from build123d import *

# Parameters (mm, degrees)
F0_W     = 90
F0_H     = 60
F0_R     = 2.15
F1_DEPTH = 60
F2_R     = 1.5
F3_DEPTH = 60
F4_W     = 50
F4_H     = 50
F5_DEPTH = 90


with BuildPart() as f1:
    # F0 (on Top) → F1 (new body)
    with BuildSketch(Plane.XY):
        Rectangle(F0_W, F0_H)
        with Locations((-39.25, -13)):
            Circle(F0_R, mode=Mode.SUBTRACT)
        with Locations((-8.75, -13)):
            Circle(F0_R, mode=Mode.SUBTRACT)
        with Locations((8.75, -13)):
            Circle(F0_R, mode=Mode.SUBTRACT)
        with Locations((39.25, -13)):
            Circle(F0_R, mode=Mode.SUBTRACT)
        with Locations((-39.25, 13)):
            Circle(F0_R, mode=Mode.SUBTRACT)
        with Locations((-8.75, 13)):
            Circle(F0_R, mode=Mode.SUBTRACT)
        with Locations((8.75, 13)):
            Circle(F0_R, mode=Mode.SUBTRACT)
        with Locations((39.25, 13)):
            Circle(F0_R, mode=Mode.SUBTRACT)
    extrude(amount=-F1_DEPTH)

    # F2 (on face) → F3 (cut)
    with BuildSketch(Plane.XY):
        Circle(F2_R)
    extrude(amount=-F3_DEPTH, mode=Mode.SUBTRACT)

    # F4 (on face) → F5 (cut)
    with BuildSketch(Plane.YZ.offset(45)):
        with Locations((0, -30)):
            Rectangle(F4_W, F4_H)
    extrude(amount=-F5_DEPTH, mode=Mode.SUBTRACT)


solid = f1.part
Can you work these out from the model? Positions are in its coordinate system, mm. A direction names the side the tool comes from. Round coordinates to 2 decimals unless told otherwise and drop trailing zeros. Write each loop counter-clockwise with the first axis right and the second up, starting at its lowest first coordinate (ties: lowest second). Pieces come first, ordered by that corner, then holes. Notation, with made-up numbers: (35.5, -30.75) -> (93.5, -30.75) arc R12 ccw to (93.5, -26.75) -> close; hole circle Ø6 at (7, -34). An arc over 180 degrees is marked (long way). Use one line per item in the form item = value. Start each with the question number.
Q1. Imagine slicing it at D-D (y = 0). Please give me the cut outline in (x, z), then the cut area to 3 significant figures.
Q2. Imagine slicing it at B-B (x = 0). Please give me the cut outline in (y, z).
Q3. Which directions (+Z, -Z, +X, -X, +Y, -Y) give clear straight access to the entire face, cutting with the end or side of a thin tool? Please do faces 4 (the face through (1, 5, -55)), 5 (the face through (-1, 30, -30)).
Q4. Imagine slicing it at C-C (z = -48). Please give me the cut outline in (x, y), then the cut area to 3 significant figures.
Q5. Imagine slicing it at A-A (x = 39.25). Please give me the cut outline in (y, z).
Q6. If I drill on probe 1 along Y at (x, z) = (-39, -2); probe 2 along Z at (x, y) = (20.5, -21.5); probe 3 along Y at (x, z) = (41.5, -22), over which ranges is the centre line in solid material (lowest first)? Write a range as [from, to].
Q7. I'm going to push flat-ended pins straight in: P1, Ø5, axis at x = -8.75, y = -13, coming from the +Z side; P2, Ø4, axis at x = -39.25, y = 13, coming from the +Z side. Where does each tip first touch, or does it pass through?
Q8. We'd pull the mould along X, two halves only. Please class faces 1 (the face through (-1, 7, 0)), 2 (the face through (45, -27, -30)), 3 (the face through (41.236, -13.823, -57.465)): +X half, -X half, draft (parallel to the pull), parting line (faces both ways), or undercut.
Worked out:
q1.outline = (-45, -60) -> (-1.5, -60) -> (-1.5, -55) -> (-45, -55) -> close; (-45, -5) -> (-1.5, -5) -> (-1.5, 0) -> (-45, 0) -> close; (1.5, -60) -> (45, -60) -> (45, -55) -> (1.5, -55) -> close; (1.5, -5) -> (45, -5) -> (45, 0) -> (1.5, 0) -> close
q1.area = 870 mm^2
q2.outline = (-30, -60) -> (-1.5, -60) -> (-1.5, -55) -> (-25, -55) -> (-25, -5) -> (-1.5, -5) -> (-1.5, 0) -> (-30, 0) -> close; (1.5, -60) -> (30, -60) -> (30, 0) -> (1.5, 0) -> (1.5, -5) -> (25, -5) -> (25, -55) -> (1.5, -55) -> close
q3.face_4 = +X, -X
q3.face_5 = +Z, -Z, +X, -X, +Y
q4.outline = (-45, -30) -> (45, -30) -> (45, -25) -> (-45, -25) -> close; (-45, 25) -> (45, 25) -> (45, 30) -> (-45, 30) -> close
q4.area = 900 mm^2
q5.outline = (-30, -60) -> (-15.15, -60) -> (-15.15, -55) -> (-25, -55) -> (-25, -5) -> (-15.15, -5) -> (-15.15, 0) -> (-30, 0) -> close; (-10.85, -60) -> (10.85, -60) -> (10.85, -55) -> (-10.85, -55) -> close; (-10.85, -5) -> (10.85, -5) -> (10.85, 0) -> (-10.85, 0) -> close; (15.15, -60) -> (30, -60) -> (30, 0) -> (15.15, 0) -> (15.15, -5) -> (25, -5) -> (25, -55) -> (15.15, -55) -> close
q6.probe_1 = [-30, -15.14], [-10.86, 10.86], [15.14, 30]
q6.probe_2 = [-60, -55], [-5, 0]
q6.probe_3 = [-30, -25], [25, 30]
q7.P1 = 0
q7.P2 = through
q8.face_1 = draft
q8.face_2 = +X half
q8.face_3 = undercut
